Here's how the part is built. I have some questions about the finished solid (model axes, mm). Round coordinates to 2 decimals unless told otherwise and drop trailing zeros. Order: outer loops, then holes, each group sorted by start corner. A loop starts at its lowest first (then second) coordinate and runs counter-clockwise, first axis right, second up. Notation, with made-up numbers: (15, 52) - (55, 52) arc R13 ccw to (55, 63) - close; hole circle Ø6 at (79, -16.5). An arc over 180 degrees is marked (long way). One line per item, written item: value.
Autodesk Inventor part; units mm, degrees
ref_plane "YZ Plane" through (0, 0, 0) normal (1, 0, 0) x (0, 1, 0)
ref_plane "XZ Plane" through (0, 0, 0) normal (0, 1, 0) x (-1, 0, 0)
ref_plane "XY Plane" through (0, 0, 0) normal (0, 0, 1) x (1, 0, 0)
sketch "スケッチ1" plane through (0, 0, 0) normal (0, 0, 1) x (1, 0, 0)
  line L0 (0, 0) -> (30, 0)
  line L1 (30, 0) -> (30, 30)
  line L2 (30, 30) -> (0, 30)
  line L3 (0, 30) -> (0, 0)
  dimension "d0" = 30
  dimension "d1" = 30
extrude "押し出し1" add sketch "スケッチ1" along normal blind 2
sketch "スケッチ2" plane through (0, 0, 2) normal (0, 0, 1) x (1, 0, 0)
  line L0 (30, 0) -> (30, 30)
  line L1 (30, 30) -> (0, 30)
  line L2 (0, 30) -> (0, 0)
  line L3 (0, 0) -> (30, 0)
  point P0 (25, 25)
  point P1 (5, 25)
  point P2 (5, 5)
  point P3 (25, 5)
  dimension "d4" = 5
  dimension "d5" = 5
  dimension "d6" = 5
  dimension "d7" = 5
  dimension "d8" = 5
  dimension "d9" = 5
  dimension "d10" = 5
  dimension "d11" = 5
hole "穴1" at (25, 25, 2) at (5, 25, 2) at (5, 5, 2) at (25, 5, 2) direction (0, 0, -1) diameter 3.5 end through all
sketch "スケッチ3" plane through (0, 0, 2) normal (0, 0, 1) x (1, 0, 0)
  line L0 (30, 0) -> (30, 30)
  line L1 (30, 30) -> (0, 30)
  point P0 (0, 0)
  point P1 (15, 15)
  dimension "d19" = 15
  dimension "d20" = 15
hole "穴2" at (15, 15, 2) direction (0, 0, -1) diameter 6.5 end through all
properties part number "3SR15_ポテンショメータ固定パーツ"
Q1. If we section it at B-B, the plane y = 15: Please give me the cut outline in (x, z).
Results list:
outline: (0, 0) - (11.75, 0) - (11.75, 2) - (0, 2) - close; (18.25, 0) - (30, 0) - (30, 2) - (18.25, 2) - close
Q2. If I drill on line 1 along Y through (x, z) = (5, 0.7); line 2 along Y through (x, z) = (12.5, 0.2), over which ranges is the centre line in solid material (lowest first)?
Results list:
line 1: 0 to 3.25, 6.75 to 23.25, 26.75 to 30
line 2: 0 to 12.92, 17.08 to 30
Q3. We'd pull the mould along Y, two halves only. Please class faces 1 (the flat face through (15, 0, 1)), 2 (the flat face through (11, 15, 2)), 3 (the cylindrical face through (4.92, 26.75, 0.99)): released by +Y, released by -Y, zero draft, split by the parting line, or undercut.
Results list:
face 1: released by -Y
face 2: zero draft
face 3: undercut
Q4. Will this pin go through, and if not, where does the flat tip stop? pin 1 (3 mm diameter, centred on x = 25, y = 25, fed in from +Z).
Results list:
pin 1: through
Q5. If we section it at A-A, the plane z = 0.8: Please give me the cut outline in (x, y), then the cut area to 3 significant figures.
Results list:
outline: (0, 0) - (30, 0) - (30, 30) - (0, 30) - close; hole circle Ø3.5 at (5, 5); hole circle Ø3.5 at (5, 25); hole circle Ø6.5 at (15, 15); hole circle Ø3.5 at (25, 5); hole circle Ø3.5 at (25, 25)
area: 828 mm²
Q6. If we section it at C-C, the plane x = 5: Please give me the cut outline in (y, z).
Results list:
outline: (0, 0) - (3.25, 0) - (3.25, 2) - (0, 2) - close; (6.75, 0) - (23.25, 0) - (23.25, 2) - (6.75, 2) - close; (26.75, 0) - (30, 0) - (30, 2) - (26.75, 2) - close
